Input: dimensioned drawing with shaded views. Units: mm. Origin: part minimum x, y, z. A direction names the side the tool comes from. Round coordinates to 2 decimals unless told otherwise and drop trailing zeros. Loops run counter-clockwise (first coordinate to the right, second up) from the corner with the lowest first, then second, coordinate; pieces in that order, holes last. Notation, with made-up numbers: M 75,-24 L 90,-24 A21 ccw 90,-18 Z; hole C 55,15 d2. An arc over 180 degrees is marked long. Return JSON: item names as keys, results as strings.
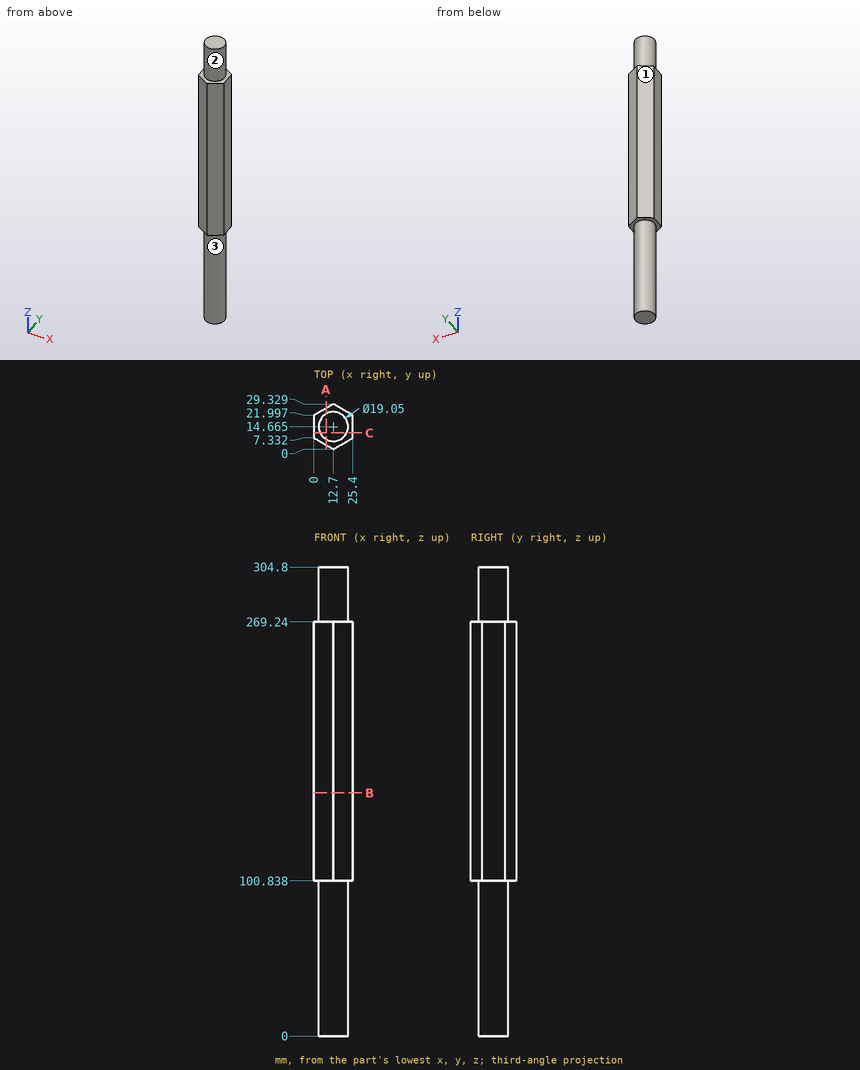
Q1. Section query C-C (y = 10.5). Output: boundary loops of the cut face in (x, z), plus the area to 3 significant figures.
Determined:
{"outline": "M 0,100.84 L 4.13,100.84 L 4.13,0 L 21.27,0 L 21.27,100.84 L 25.4,100.84 L 25.4,269.24 L 21.27,269.24 L 21.27,304.8 L 4.13,304.8 L 4.13,269.24 L 0,269.24 Z", "area": "6,610 mm^2"}
Q2. Reachability of the marked faces 1, 2 and 3 from +Z, -Z, +X, -X, +Y, -Y: full face, straight path, thin tool, end or side. Return the list, or none.
Determined:
{"face 1": "+Z, -Z, -X, +Y", "face 2": "+Z", "face 3": "-Z"}
Q3. Pin query (flat end, axial travel): pin 1 (10 mm diameter, centred on x = 7, z = 41.5, fed in from +Y); pin 2 (6 mm diameter, centred on x = 12, z = 64, fed in from -Y); pin 3 (5 mm diameter, centred on x = 7.5, z = 192.5, fed in from -Y). Return the tip coordinate at first contact, or that it passes through.
Determined:
{"pin 1": "stops at y = 24.16", "pin 2": "stops at y = 5.14", "pin 3": "stops at y = 1.56"}
Q4. Section query A-A (x = 8). Output: boundary loops of the cut face in (y, z).
Determined:
{"outline": "M 2.71,100.84 L 6.38,100.84 L 6.38,0 L 22.95,0 L 22.95,100.84 L 26.62,100.84 L 26.62,269.24 L 22.95,269.24 L 22.95,304.8 L 6.38,304.8 L 6.38,269.24 L 2.71,269.24 Z"}
Q5. Material intervals for L1, parallel to Z at x = 4.25, y = 21; L2, parallel to Y at x = 14.5, z = 281.5; L3, parallel to Y at x = 21, z = 58 (1 decimal), sorted ascending.
Determined:
{"L1": "z = 100.84 to 269.24", "L2": "y = 5.31 to 24.02", "L3": "y = 10 to 19.3"}
Q6. Section query B-B (z = 158). Output: boundary loops of the cut face in (x, y).
Determined:
{"outline": "M 0,7.33 L 12.7,0 L 25.4,7.33 L 25.4,22 L 12.7,29.33 L 0,22 Z"}
